from build123d import *

# Parameters (mm, degrees)
EXTRUDE_1_DEPTH = 4


with BuildPart() as part:
    # 草圖1 → 填料-伸長1 (new body)
    with BuildSketch(Plane.XY):
        with BuildLine():
            Line((0, 0), (3, 0))
            Line((3, 0), (3, 1))
            ThreePointArc((3, 1), (3.292893219, 1.707106781), (4, 2))
            Line((4, 2), (6, 2))
            Line((6, 2), (6, 3))
            Line((6, 3), (3, 3))
            ThreePointArc((3, 3), (2.292893219, 3.292893219), (2, 4))
            Line((2, 4), (2, 5))
            Line((2, 5), (1, 5))
            Line((1, 5), (1, 4))
            Line((1, 4), (-1, 4))
            Line((-1, 4), (-1, 1))
            Line((-1, 1), (0, 1))
            Line((0, 1), (0, 0))
        make_face()
    extrude(amount=EXTRUDE_1_DEPTH)


solid = part.part
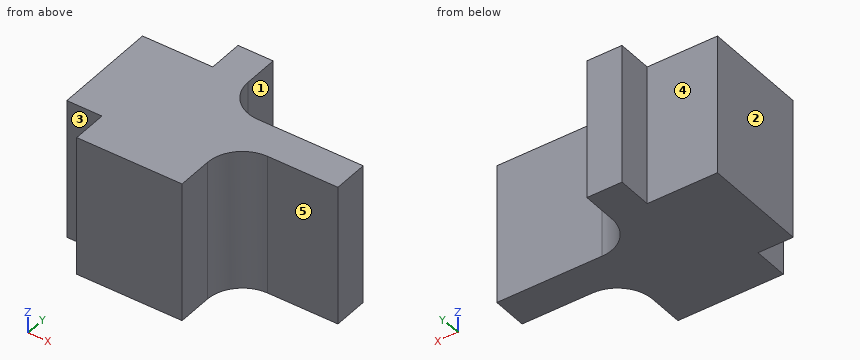
The listing builds one solid part. Answer for the finished solid, in the listing's coordinates (mm). Face numbers are marked on the shaded views. A direction names the side the tool comes from. Round coordinates to 2 decimals unless told otherwise and drop trailing zeros. Write each loop counter-clockwise with the first axis right and the second up, starting at its lowest first coordinate (ties: lowest second). Pieces come first, ordered by that corner, then holes. Notation, with made-up numbers: M 32,27 L 69,27 A20 ccw 69,33 Z; hole C 10.25,63.25 d11. An arc over 180 degrees is marked long. Write each question's results on one line, items separated by ' | '. Start each with the question number.
Item 1: Given pin 1 Ø1.1 at (x, z) = (-0.5, 2.5) entering from -Y; pin 2 Ø0.5 at (y, z) = (0.5, 2) entering from +X; pin 3 Ø0.9 at (x, z) = (4.5, 2.5) entering from +Y; pin 4 Ø0.8 at (y, z) = (4.5, 2.5) entering from -X, each flat-ended and moving along its own axis, determine where each tip first touches the part or whether it passes through.
Item 2: Find section A-A on z = 3.4. Write down the section's boundary in (x, y).
Item 3: Straight lines are drawn through the part: probe 1 along Y at (x, z) = (5.5, 2.4); probe 2 along Y at (x, z) = (0.5, 2.45); probe 3 along X at (y, z) = (4.25, 0.95). For each, find the intervals that lie inside material, in ascending order.
Item 4: Find section C-C on y = 0.45. Write down the section's boundary in (x, z).
Item 5: Which of the six approach directions +Z, -Z, +X, -X, +Y, -Y give full straight-line access (tool end or side, diameter ignored) to the marked faces 1, 2, 3, 4 and 5?
Item 6: Find section B-B on x = -0.5. Write down the section's boundary in (y, z).
Answer block:
1) pin 1: stops at y = 0 | pin 2: stops at x = 3 | pin 3: stops at y = 3 | pin 4: stops at x = 1
2) outline: M -1,1 L 0,1 L 0,0 L 3,0 L 3,1 A1 cw 4,2 L 6,2 L 6,3 L 3,3 A1 cw 2,4 L 2,5 L 1,5 L 1,4 L -1,4 Z
3) probe 1: y = 2 to 3 | probe 2: y = 0 to 4 | probe 3: x = 1 to 2
4) outline: M 0,0 L 3,0 L 3,4 L 0,4 Z
5) face 1: +Z, -Z, +X, +Y | face 2: +Z, -Z, -X, +Y, -Y | face 3: +Z, -Z, -X, -Y | face 4: +Z, -Z, -X, +Y | face 5: +Z, -Z, +X, -Y
6) outline: M 1,0 L 4,0 L 4,4 L 1,4 Z
